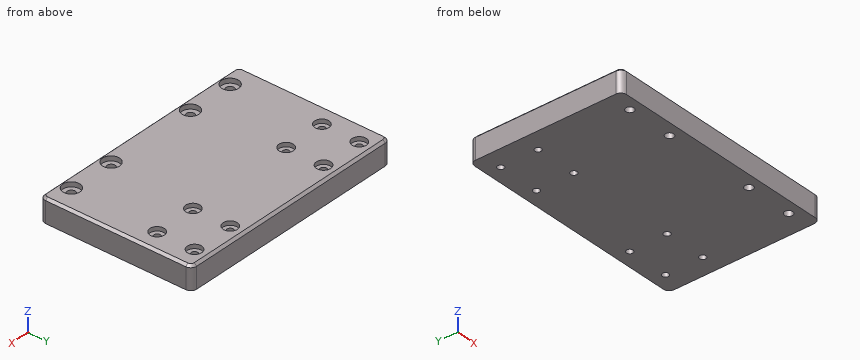
```python
from build123d import *

# Parameters (mm, degrees)
SKETCH1_W                               = 200
SKETCH1_H                               = 130
BOSS_EXTRUDE1_DEPTH                     = 20
FILLET1_R                               = 5
CBORE_FOR_M6_HEX_HEAD_BOLT2_AT_2_COUNT  = 2
CBORE_FOR_M6_HEX_HEAD_BOLT2_AT_2_PITCH  = 40
CBORE_FOR_M6_HEX_HEAD_BOLT2_AT_3_COUNT  = 2
CBORE_FOR_M6_HEX_HEAD_BOLT2_AT_3_PITCH  = 120
CBORE_FOR_M6_HEX_HEAD_BOLT2_AT_4_COUNT  = 2
CBORE_FOR_M6_HEX_HEAD_BOLT2_AT_4_PITCH  = 160
CBORE_FOR_M5_HEX_HEAD_BOLT1_D           = 5.5
CBORE_FOR_M5_HEX_HEAD_BOLT1_CBORE_D     = 12.238
CBORE_FOR_M5_HEX_HEAD_BOLT1_CBORE_DEPTH = 3.5
CHAMFER1_SIZE                           = 2


with BuildPart() as part:
    # Sketch1 → Boss-Extrude1 (new body)
    with BuildSketch(Plane.XY):
        with Locations((100, 65)):
            Rectangle(SKETCH1_W, SKETCH1_H)
    extrude(amount=BOSS_EXTRUDE1_DEPTH)

    # Fillet1
    fillet1_edges = [part.edges().sort_by_distance(p)[0] for p in [
        (0, 130, 10),
        (200, 130, 10),
        (200, 0, 10),
        (0, 0, 10),
    ]]
    fillet(fillet1_edges, radius=FILLET1_R)

    # Sketch17 → CBORE for M6 Hex Head Bolt2 (revolve, cut)
    with BuildSketch(Plane(origin=(20, 10, 20), x_dir=(0, -1, 0), z_dir=(1, 0, 0))):
        Polygon((0, 0), (0, 20), (3.5, 20), (3.5, 4), (7.2735, 4), (7.2735, 0.025), (7.2985, 0), align=None)
    cbore_for_m6_hex_head_bolt2 = revolve(axis=Axis((20, 10, 26.35), (0, 0, -1)), mode=Mode.SUBTRACT)

    # CBORE for M6 Hex Head Bolt2 at 2: CBORE for M6 Hex Head Bolt2 ×2
    with Locations(*[(i * CBORE_FOR_M6_HEX_HEAD_BOLT2_AT_2_PITCH, 0, 0) for i in range(1, CBORE_FOR_M6_HEX_HEAD_BOLT2_AT_2_COUNT)]):
        add(cbore_for_m6_hex_head_bolt2, mode=Mode.SUBTRACT)

    # CBORE for M6 Hex Head Bolt2 at 3: CBORE for M6 Hex Head Bolt2 ×2
    with Locations(*[(i * CBORE_FOR_M6_HEX_HEAD_BOLT2_AT_3_PITCH, 0, 0) for i in range(1, CBORE_FOR_M6_HEX_HEAD_BOLT2_AT_3_COUNT)]):
        add(cbore_for_m6_hex_head_bolt2, mode=Mode.SUBTRACT)

    # CBORE for M6 Hex Head Bolt2 at 4: CBORE for M6 Hex Head Bolt2 ×2
    with Locations(*[(i * CBORE_FOR_M6_HEX_HEAD_BOLT2_AT_4_PITCH, 0, 0) for i in range(1, CBORE_FOR_M6_HEX_HEAD_BOLT2_AT_4_COUNT)]):
        add(cbore_for_m6_hex_head_bolt2, mode=Mode.SUBTRACT)

    # CBORE for M5 Hex Head Bolt1 (through all)
    with Locations(Plane.XY.offset(20)):
        with Locations((17, 118), (53, 118), (53, 86), (17, 86), (183, 118), (183, 86), (147, 118), (147, 86)):
            CounterBoreHole(CBORE_FOR_M5_HEX_HEAD_BOLT1_D / 2, CBORE_FOR_M5_HEX_HEAD_BOLT1_CBORE_D / 2, CBORE_FOR_M5_HEX_HEAD_BOLT1_CBORE_DEPTH)

    # Chamfer1
    chamfer1_edges = [part.edges().sort_by_distance(p)[0] for p in [
        (100, 130, 20),
        (200, 65, 20),
        (0, 65, 20),
        (100, 0, 20),
        (1.464466094, 128.535533906, 20),
        (1.464466094, 1.464466094, 20),
        (198.535533906, 1.464466094, 20),
        (198.535533906, 128.535533906, 20),
    ]]
    chamfer(chamfer1_edges, length=CHAMFER1_SIZE)


solid = part.part
```
Geometry check sheet. Reference: the model listing, model coordinates, mm. Coordinates: 2 decimals unless noted, no trailing zeros. Use CSV: the item, a comma, the result in double quotes. Start each with the question number.
Item 1: Depth check by flat-ended pin: pin 1 Ø16 at (x, y) = (136.5, 13) entering from +Z; pin 2 Ø10 at (x, y) = (147, 118) entering from +Z; pin 3 Ø7.5 at (x, y) = (19, 8) entering from +Z. Enter the tip coordinate at first touch or a pass-through.
Item 2: Thickness scan on line 1 (X direction, y = 10, z = 11.5); line 2 (Y direction, x = 140, z = 16.9); line 3 (X direction, y = 8, z = 8.75). Record the ranges inside material, lowest first.
Item 3: Cross-section at A-A, the plane y = 86. State how many separate pieces and enclosed holes the cut face has, plus the area to 3 significant figures.
Answers:
1,pin 1,"z = 20"
1,pin 2,"z = 16.5"
1,pin 3,"z = 16"
2,line 1,"0 to 16.5, 23.5 to 56.5, 63.5 to 136.5, 143.5 to 176.5, 183.5 to 200"
2,line 2,"0 to 2.73, 17.27 to 130"
2,line 3,"0 to 17.13, 22.87 to 57.13, 62.87 to 137.13, 142.87 to 177.13, 182.87 to 200"
3,separate pieces,"5"
3,enclosed holes,"0"
3,area,"3,460 mm^2"
